The listing builds one solid part. Answer for the finished solid, in the listing's coordinates (mm). A direction names the side the tool comes from. Coordinates: 2 decimals unless noted, no trailing zeros. Order: outer loops, then holes, each group sorted by start corner. A loop starts at its lowest first (then second) coordinate and runs counter-clockwise, first axis right, second up.
from build123d import *

# Parameters (mm, degrees)
BOSS_EXTRUDE1_DEPTH                            = 75
SKETCH5_R                                      = 1.75
CUT_EXTRUDE1_DEPTH                             = 2
CSK_FOR_0_FLAT_HEAD_MACHINE_SCREW2_D           = 1.778
CSK_FOR_0_FLAT_HEAD_MACHINE_SCREW2_DEPTH       = 3.302
CSK_FOR_0_FLAT_HEAD_MACHINE_SCREW2_CSINK_D     = 3.0226
CSK_FOR_0_FLAT_HEAD_MACHINE_SCREW2_CSINK_ANGLE = 82
CSK_FOR_0_FLAT_HEAD_MACHINE_SCREW2_TIP         = 0.53416509
CHAMFER1_SIZE                                  = 3
SKETCH6_W                                      = 1.5
SKETCH6_H                                      = 5
BOSS_EXTRUDE2_DEPTH                            = 5
CSK_FOR_0_FLAT_HEAD_MACHINE_SCREW1_D           = 1.778
CSK_FOR_0_FLAT_HEAD_MACHINE_SCREW1_DEPTH       = 3.302
CSK_FOR_0_FLAT_HEAD_MACHINE_SCREW1_CSINK_D     = 3.0226
CSK_FOR_0_FLAT_HEAD_MACHINE_SCREW1_CSINK_ANGLE = 82
CSK_FOR_0_FLAT_HEAD_MACHINE_SCREW1_TIP         = 0.53416509


with BuildPart() as part:
    # Sketch1 → Boss-Extrude1 (new body)
    with BuildSketch(Plane.XY):
        Polygon((-2, -3), (2, -3), (2, -0.5), (0, -0.5), (0, 0.5), (2, 0.5), (2, 3), (-2, 3), align=None)
    extrude(amount=BOSS_EXTRUDE1_DEPTH)

    # Sketch5 → Cut-Extrude1 (cut)
    with BuildSketch(Plane(origin=(2, 0, 0), x_dir=(0, 0, -1), z_dir=(1, 0, 0))):
        with Locations((-65, 0)):
            Circle(SKETCH5_R)
        with Locations((-46.66667, 0)):
            Circle(SKETCH5_R)
        with Locations((-28.33334, 0)):
            Circle(SKETCH5_R)
        with Locations((-10.00001, 0)):
            Circle(SKETCH5_R)
    extrude(amount=-CUT_EXTRUDE1_DEPTH, mode=Mode.SUBTRACT)

    # CSK for #0 Flat Head Machine Screw2
    with Locations(Plane(origin=(0, 0, 0), x_dir=(0, 0, -1), z_dir=(1, 0, 0))):
        with Locations((-65, 0), (-10.00001, 0), (-46.66667, 0), (-28.33334, 0)):
            CounterSinkHole(CSK_FOR_0_FLAT_HEAD_MACHINE_SCREW2_D / 2, CSK_FOR_0_FLAT_HEAD_MACHINE_SCREW2_CSINK_D / 2, depth=CSK_FOR_0_FLAT_HEAD_MACHINE_SCREW2_DEPTH, counter_sink_angle=CSK_FOR_0_FLAT_HEAD_MACHINE_SCREW2_CSINK_ANGLE)
            with Locations((0, 0, -(CSK_FOR_0_FLAT_HEAD_MACHINE_SCREW2_DEPTH + CSK_FOR_0_FLAT_HEAD_MACHINE_SCREW2_TIP / 2))):  # 118° drill point
                Cone(0, CSK_FOR_0_FLAT_HEAD_MACHINE_SCREW2_D / 2, CSK_FOR_0_FLAT_HEAD_MACHINE_SCREW2_TIP, mode=Mode.SUBTRACT)

    # Chamfer1
    # the kernel refuses this chamfer: 3 mm, written as the material it takes off along each edge
    with BuildSketch(Plane(origin=(2, -3, -7.715048964), x_dir=(-0.9996219169112968, -0.027495876610586348, 0), z_dir=(0, 0, 1))) as chamfer1_piece_1:
        Polygon((CHAMFER1_SIZE * 0.999621916911, -CHAMFER1_SIZE * 0.0274958766106), (-CHAMFER1_SIZE * 0.0274958766106, -CHAMFER1_SIZE * 0.999621916911), (0, 0), align=None)
    extrude(amount=90.430097928, mode=Mode.SUBTRACT)
    with BuildSketch(Plane(origin=(2, 3, -7.715048964), x_dir=(-0.9996219169112968, 0.027495876610586348, 0), z_dir=(0, 0, 1))) as chamfer1_piece_2:
        Polygon((CHAMFER1_SIZE * 0.999621916911, CHAMFER1_SIZE * 0.0274958766106), (-CHAMFER1_SIZE * 0.0274958766106, CHAMFER1_SIZE * 0.999621916911), (0, 0), align=None)
    extrude(amount=90.430097928, mode=Mode.SUBTRACT)

    # Sketch6 → Boss-Extrude2 (add)
    with BuildSketch(Plane.XY.offset(75)):
        Polygon((2, 0.5), (2, 3), (0.5, 3), (-2, 3), (-2, -3), (2, -3), (2, -0.5), (0, -0.5), (0, 0.5), align=None)
        with Locations((1.25, 5.5)):
            Rectangle(SKETCH6_W, SKETCH6_H)
    extrude(amount=BOSS_EXTRUDE2_DEPTH)

    # CSK for #0 Flat Head Machine Screw1
    with Locations(Plane(origin=(2, 0, 0), x_dir=(0, 0, -1), z_dir=(1, 0, 0))):
        with Locations((-77.5, 5.5)):
            CounterSinkHole(CSK_FOR_0_FLAT_HEAD_MACHINE_SCREW1_D / 2, CSK_FOR_0_FLAT_HEAD_MACHINE_SCREW1_CSINK_D / 2, depth=CSK_FOR_0_FLAT_HEAD_MACHINE_SCREW1_DEPTH, counter_sink_angle=CSK_FOR_0_FLAT_HEAD_MACHINE_SCREW1_CSINK_ANGLE)
            with Locations((0, 0, -(CSK_FOR_0_FLAT_HEAD_MACHINE_SCREW1_DEPTH + CSK_FOR_0_FLAT_HEAD_MACHINE_SCREW1_TIP / 2))):  # 118° drill point
                Cone(0, CSK_FOR_0_FLAT_HEAD_MACHINE_SCREW1_D / 2, CSK_FOR_0_FLAT_HEAD_MACHINE_SCREW1_TIP, mode=Mode.SUBTRACT)


solid = part.part
1) Section C-C (z = 18) is taken. Give the vertices of the cut face in (x, y).
2) Consider L1, parallel to Y at x = 0.7, z = 77.5; L2, parallel to Z at x = -1.05, y = 0; L3, parallel to Z at x = 0.7, y = 5.5. Determine where each line is inside the solid, lowest interval first.
3) Each of these flat-tipped pins is pushed along its axis until it touches: P1, Ø0.8, axis at x = 0.5, z = 3.5, coming from the -Y side; P2, Ø0.6, axis at x = 1.5, z = 74, coming from the +Y side; P3, Ø1.1, axis at y = 0, z = 28.33, coming from the +X side; P4, Ø2, axis at x = 1, z = 27.5, coming from the +Y side. Where does it stop, or does it pass through?
4) Determine the mould class of faces 4 (the face through (0.89, 5.16, 78.32)), 5 (the face through (-1.3, 3, 39.4)), 6 (the face through (-1.2, -3, 45.7)) for opening direction Y: released by +Y, released by -Y, zero draft, split by the parting line, or undercut.
5) A tool of negligible diameter and unlimited length cuts with its end or side. For faces 1 (the face through (1, 0.5, 19)), 2 (the face through (0, 0, 43)), 3 (the face through (-1.367, 0.267, 65.848)), from which of +Z, -Z, +X, -X, +Y, -Y can it reach the whole face along a straight path? Write none if from no direction.
6) Section B-B (y = 5.5) is taken. Give the vertices of the cut face in (x, z).
7) Section A-A (z = 65) is taken. Give the vertices of the cut face in (x, y), then the cut area to 3 significant figures.
Filled sheet:
1. outline: (-2, -3) - (-1, -3) - (1.5, -0.5) - (0, -0.5) - (0, 0.5) - (1.5, 0.5) - (-1, 3) - (-2, 3) - close
2. L1: y = -3 to -0.5, 0.5 to 4.61, 6.39 to 8
2. L2: z = 0 to 9.11, 10.89 to 27.44, 29.22 to 45.78, 47.56 to 64.11, 65.89 to 80
2. L3: z = 75 to 76.61, 78.39 to 80
3. P1: stops at y = -1.9
3. P2: stops at y = 0.8
3. P3: passes through
3. P4: stops at y = 2
4. face 4: undercut
4. face 5: released by +Y
4. face 6: released by -Y
5. face 1: +Z, -Z, +X
5. face 2: +X
5. face 3: +X, -X
6. outline: (0.5, 75) - (2, 75) - (2, 75.99) - (1.28, 76.61) - (0.5, 76.61) - close; (0.5, 78.39) - (1.28, 78.39) - (2, 79.01) - (2, 80) - (0.5, 80) - close
7. outline: (-2, -3) - (-1, -3) - (0.25, -1.75) - (0, -1.75) - (0, -1.51) - (-0.72, -0.89) - (-2, -0.89) - close; (-2, 0.89) - (-0.72, 0.89) - (0, 1.51) - (0, 1.75) - (0.25, 1.75) - (-1, 3) - (-2, 3) - close
7. area: 7.06 mm2
